Could you check a few things on this drawing? It's one solid part, dimensions in mm from its lowest x, y, z. Give positions to 0.01 mm unless a question says otherwise; leave off trailing zeros. Write each loop counter-clockwise with the first axis right and the second up, starting at its lowest first coordinate (ties: lowest second). Pieces come first, ordered by that corner, then holes.
1. If I drill on probe 1 along Y at (x, z) = (2.5, 1.1); probe 2 along Y at (x, z) = (9.5, 1.85); probe 3 along X at (y, z) = (5, 0.25), over which ranges is the centre line in solid material (lowest first)?
2. Suppose I cut it at B-B (x = 2.5). Please give me the cut outline in (y, z).
3. Suppose I cut it at A-A (z = 1.45). Please give me the cut outline in (x, y), and give its area (3 significant figures).
4. Suppose I cut it at C-C (y = 2.5). Please give me the cut outline in (x, z).
5. I'm going to push flat-ended pins straight in: pin 1 (2.5 mm diameter, centred on x = 9.62, y = 8, fed in from -Z); pin 2 (4 mm diameter, centred on x = 36.5, y = 8, fed in from -Z). Where does each tip first touch, or does it pass through?
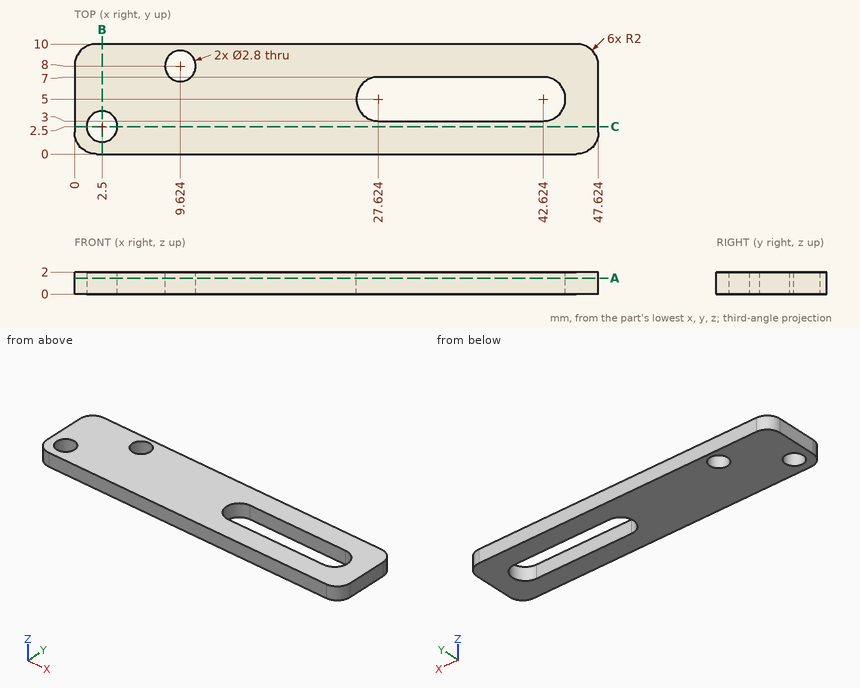
Checks:
1. probe 1: y = 0 to 1.1, 3.9 to 10
1. probe 2: y = 0 to 6.61, 9.39 to 10
1. probe 3: x = 0 to 25.62, 44.62 to 47.62
2. outline: (0, 0) - (1.1, 0) - (1.1, 2) - (0, 2) - close; (3.9, 0) - (10, 0) - (10, 2) - (3.9, 2) - close
3. outline: (0, 2) arc R2 ccw to (2, 0) - (45.62, 0) arc R2 ccw to (47.62, 2) - (47.62, 8) arc R2 ccw to (45.62, 10) - (2, 10) arc R2 ccw to (0, 8) - close; hole circle Ø2.8 at (2.5, 2.5); hole circle Ø2.8 at (9.62, 8); hole (27.62, 3) - (42.62, 3) arc R2 ccw to (42.62, 7) - (27.62, 7) arc R2 ccw to start
3. area: 388 mm2
4. outline: (0, 0) - (1.1, 0) - (1.1, 2) - (0, 2) - close; (3.9, 0) - (47.62, 0) - (47.62, 2) - (3.9, 2) - close
5. pin 1: passes through
5. pin 2: stops at z = 0
